Autodesk Inventor part; units mm, degrees
ref_plane "YZ Plane" through (0, 0, 0) normal (1, 0, 0) x (0, 1, 0)
ref_plane "XZ Plane" through (0, 0, 0) normal (0, 1, 0) x (-1, 0, 0)
ref_plane "XY Plane" through (0, 0, 0) normal (0, 0, 1) x (1, 0, 0)
sketch "Sketch1" plane through (0, 0, 0) normal (1, 0, 0) x (0, 1, 0)
  circle A0 centre (0, 0) radius 2.5
  arc A1 (0, 4) -> (0, -4) centre (0, 0) ccw
  line L0 (0, 4) -> (100, 4)
  line L1 (100, -4) -> (0, -4)
  arc A2 (100, -4) -> (100, 4) centre (100, 0) ccw
  circle A3 centre (100, 0) radius 2.5
  dimension "d0" = 5
  dimension "d1" = 8
  dimension "d3" = 100
  dimension "d4" = 8
  dimension "d5" = 5
extrude "Extrusion1" add sketch "Sketch1" along normal blind 10
ref_plane "Work Plane1" through (5, 0, 0) normal (1, 0, 0) x (0, 0, -1)
sketch "Sketch2" plane through (5, 0, 0) normal (1, 0, 0) x (0, 0, -1)
  circle A0 centre (0, 100) radius 2.5
  arc A1 (4, 100) -> (-4, 100) centre (0, 100) ccw
  line L0 (0, 104) -> (5, 104)
  line L1 (5, 104) -> (-5, 104)
  line L2 (-5, 104) -> (-5, 96)
  line L3 (-5, 96) -> (5, 96)
  line L4 (5, 96) -> (5, 104)
  point P0 (0, 0)
  dimension "d9" = 5
  dimension "d10" = 10
  dimension "d11" = 8
extrude "Extrusion2" cut sketch "Sketch2" along normal mid plane 5
sketch "Sketch4" plane through (10, 0, 0) normal (1, 0, 0) x (0, 0, -1)
  line L0 (5, -4) -> (-5, -4)
  line L1 (-5, -4) -> (-5, 4)
  line L2 (-5, 4) -> (5, 4)
  line L3 (5, 4) -> (5, -4)
  point P0 (0, 0)
  dimension "d19" = 10
  dimension "d20" = 8
extrude "Extrusion4" cut sketch "Sketch4" against normal blind 2.5
sketch "Sketch5" plane through (0, 0, 0) normal (-1, 0, 0) x (0, 0, 1)
  line L0 (5, -4) -> (-5, -4)
  line L1 (-5, -4) -> (-5, 4)
  line L2 (-5, 4) -> (5, 4)
  line L3 (5, 4) -> (5, -4)
  point P0 (0, 0)
  dimension "d23" = 10
  dimension "d24" = 8
extrude "Extrusion5" cut sketch "Sketch5" against normal blind 2.5
equation "\"d5\" = d0"
properties part number "ServoLinkage"
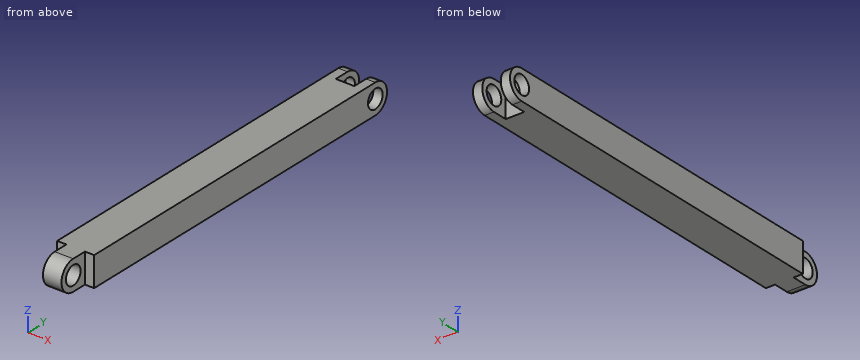
Geometry: final body of the model. Coordinates: model frame, mm. Coordinates: 2 decimals unless noted, no trailing zeros. Write each loop counter-clockwise with the first axis right and the second up, starting at its lowest first coordinate (ties: lowest second). Pieces come first, ordered by that corner, then holes. Notation, with made-up numbers: M 64,64 L 84,64 A13 cw 84,87 Z; hole C 44.25,37.5 d6. An arc over 180 degrees is marked long. Use CSV: the item, a comma, the result in double quotes. Start each with the question number.
1. Cut plane A-A on z = 0. Return the cut outline in (x, y), plus the area to 3 significant figures.
2. Cut plane B-B on x = 6. Return the cut outline in (y, z), plus the area to 4 significant figures.
3. First-contact query: P1, Ø2.5, axis at x = 5.5, z = 2, coming from the +Y side; P2, Ø4, axis at y = 100, z = 0, coming from the +X side; P3, Ø0.8, axis at x = 1, z = -1, coming from the -Y side; P4, Ø4, axis at y = 1.5, z = 1.5, coming from the -X side. Flat tips, straight axial feed; report the tip coordinate or a pass-through.
4. Ray query, probe 1 along Z at (x, y) = (5.3, 0); probe 2 along Y at (x, z) = (1, 0); probe 3 along Y at (x, z) = (4.4, 0). Return the intervals inside material, ascending.
Entries:
1,outline,"M 0,4 L 2.5,4 L 2.5,2.5 L 7.5,2.5 L 7.5,4 L 10,4 L 10,97.5 L 7.5,97.5 L 7.5,96 L 2.5,96 L 2.5,97.5 L 0,97.5 Z; M 0,102.5 L 2.5,102.5 L 2.5,104 L 0,104 Z; M 2.5,-4 L 7.5,-4 L 7.5,-2.5 L 2.5,-2.5 Z; M 7.5,102.5 L 10,102.5 L 10,104 L 7.5,104 Z"
1,area,"950 mm²"
2,outline,"M 0,-4 L 96,-4 L 96,4 L 0,4 A4 ccw Z; hole C 0,0 d5"
2,area,"773.5 mm²"
3,P1,"y = 96"
3,P2,"through"
3,P3,"y = 4"
3,P4,"x = 2.5"
4,probe 1,"-4 to -2.5, 2.5 to 4"
4,probe 2,"4 to 97.5, 102.5 to 104"
4,probe 3,"-4 to -2.5, 2.5 to 96"
